Part model, mm, in its own coordinate system. Face numbers are marked on the shaded views. A direction names the side the tool comes from. Round coordinates to 2 decimals unless told otherwise and drop trailing zeros. Write each loop counter-clockwise with the first axis right and the second up, starting at its lowest first coordinate (ties: lowest second). Pieces come first, ordered by that corner, then holes. Notation, with made-up numbers: (-29.75, 13.25) -> (-9.75, 13.25) arc R36 ccw to (-9.75, 51.25) -> close; hole circle Ø2 at (86.5, 59). An arc over 180 degrees is marked (long way). Use CSV: the item, a comma, the result in double quotes. Start each with the question number.
```python
from build123d import *

# Parameters (mm, degrees)
F1_DEPTH = 30
F2_R     = 1.5
F3_DEPTH = 25


with BuildPart() as f1:
    # F0 (on Front) → F1 (new body, symmetric)
    with BuildSketch(Plane.XZ):
        Polygon((-7.875, -2.679542), (-7.875, -18.179542), (-5, -18.179542), (-5, -12.179542), (5, -12.179542), (5, -18.179542), (7.875, -18.179542), (7.875, -2.679542), (2.65, -2.679542), (2.65, -4.679542), (-2.65, -4.679542), (-2.65, -2.679542), align=None)
    extrude(amount=F1_DEPTH, both=True)

    # F2 (on face) → F3 (cut)
    with BuildSketch(Plane.XY.offset(-4.679542)):
        with Locations((0, 4.5)):
            Circle(F2_R)
    extrude(amount=-F3_DEPTH, mode=Mode.SUBTRACT)


solid = f1.part
```
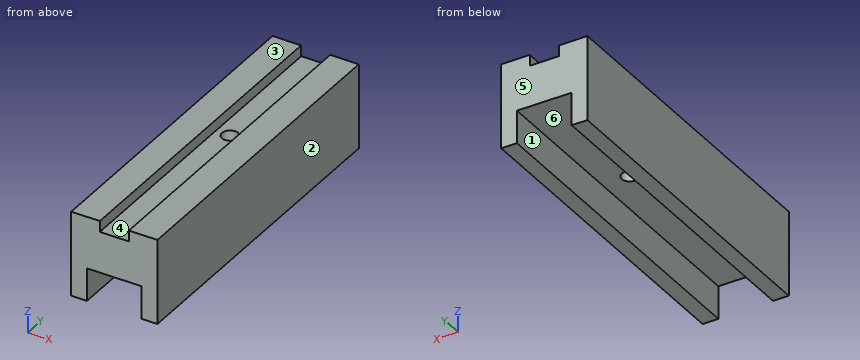
1. Band-saw the part on A-A (z = -16.25). List the corners of the cut face in (x, y) (3 decimals), then the cut area to 3 significant figures.
2. Band-saw the part on C-C (x = 0). List the corners of the cut face in (y, z).
3. Band-saw the part on D-D (x = 4). List the corners of the cut face in (y, z).
4. Drill centre lines: line 1 along X through (y, z) = (10, -13.5) (3 decimals); line 2 along Y through (x, z) = (0, -6.25); line 3 along X through (y, z) = (-24, -3.75) (3 decimals). Where is each one in solid material? Low to high. Write a range as [from, to].
5. Pull direction X, two halves, no side cores. Call the marked faces 1, 2 and 3: released by +X, released by -X, zero draft, split by the parting line, or undercut.
6. Which spindle directions (+Z, -Z, +X, -X, +Y, -Y) get a long thin tool onto all of the face, cutting with end or side? Do the marked faces 4, 5 and 6. Say none if no direction does.
7. Band-saw the part on B-B (y = 4.5). List the corners of the cut face in (x, z) (3 decimals), then the cut area to 3 significant figures.
8. Flat gauge pins, fed straight in: pin 1 (4 mm diameter, centred on x = 0, y = -5.5, fed in from +Z); pin 2 (1.5 mm diameter, centred on x = 1, z = -13.5, fed in from +Y). Where does each tip first touch, or does it go through?
Answers below:
1,outline,"(-7.875, -30) -> (-5, -30) -> (-5, 30) -> (-7.875, 30) -> close; (5, -30) -> (7.875, -30) -> (7.875, 30) -> (5, 30) -> close"
1,area,"345 mm^2"
2,outline,"(-30, -12.18) -> (3, -12.18) -> (3, -4.68) -> (-30, -4.68) -> close; (6, -12.18) -> (30, -12.18) -> (30, -4.68) -> (6, -4.68) -> close"
3,outline,"(-30, -12.18) -> (30, -12.18) -> (30, -2.68) -> (-30, -2.68) -> close"
4,line 1,"x = [-7.875, -5], [5, 7.875]"
4,line 2,"y = [-30, 3], [6, 30]"
4,line 3,"x = [-7.875, -2.65], [2.65, 7.875]"
5,face 1,"undercut"
5,face 2,"released by +X"
5,face 3,"zero draft"
6,face 4,"+Z, +Y, -Y"
6,face 5,"+Z, -Z, +X, -X, +Y"
6,face 6,"-Z, +Y, -Y"
7,outline,"(-7.875, -18.18) -> (-5, -18.18) -> (-5, -12.18) -> (-1.5, -12.18) -> (-1.5, -4.68) -> (-2.65, -4.68) -> (-2.65, -2.68) -> (-7.875, -2.68) -> close; (1.5, -12.18) -> (5, -12.18) -> (5, -18.18) -> (7.875, -18.18) -> (7.875, -2.68) -> (2.65, -2.68) -> (2.65, -4.68) -> (1.5, -4.68) -> close"
7,area,"151 mm^2"
8,pin 1,"stops at z = -4.68"
8,pin 2,"passes through"
